from build123d import *

# Parameters (mm, degrees)
F1_DEPTH = 3.175


with BuildPart() as f1:
    # F0 (on Front) → F1 (new body)
    with BuildSketch(Plane.XZ):
        with BuildLine():
            Line((-26.0459613055, 0), (-8.255, 0))
            Line((-8.255, 0), (-8.255, 3.175))
            Line((-8.255, 3.175), (8.255, 3.175))
            Line((8.255, 3.175), (8.255, 0))
            Line((8.255, 0), (20.955, 0))
            add(Edge.make_bspline(
                [(20.955, 0), (20.9736007659, 4.7706959948), (21.0039408253, 12.5522680544), (24.2599950378, 16.0448016341), (25.5707021463, 17.3285181683)],
                knots=[0, 0, 0, 0, 0.5863679016, 0.9564357243, 0.9564357243, 0.9564357243, 0.9564357243], degree=3))
            ThreePointArc((25.5707021463, 17.3285181683), (25.9142071586, 17.8340267538), (26.035, 18.4331458679))
            Line((26.035, 18.4331458679), (26.035, 30.48))
            Line((26.035, 30.48), (22.8629365507, 30.48))
            Line((22.8629365507, 30.48), (22.8629365507, 46.9999574125))
            Line((22.8629365507, 46.9999574125), (26.035, 46.9999574125))
            Line((26.035, 46.9999574125), (26.035, 53.3499574125))
            Line((26.035, 53.3499574125), (19.6908731014, 53.3499574125))
            add(Edge.make_bspline(
                [(-26.0459613055, 6.35), (-14.6993313754, 12.8784414899), (6.7793902362, 25.2365229805), (15.5524054536, 44.3388670459), (19.6908731014, 53.3499574125)],
                knots=[0, 0, 0, 0, 0.5282730572, 1, 1, 1, 1], degree=3))
            Line((-26.0459613055, 6.35), (-26.0459613055, 0))
        make_face()
    extrude(amount=F1_DEPTH)


solid = f1.part
The model under review builds one solid part; all positions refer to its coordinate system, in mm. A direction names the side the tool comes from. Coordinates: 2 decimals unless noted, no trailing zeros.
(1) Insertion check: P1, Ø1.6, axis at x = -1.5, y = -1, coming from the -Z side (3 decimals); P2, Ø8, axis at x = -18.5, z = 13.5, coming from the +Y side; P3, Ø1, axis at y = -2, z = 39, coming from the +X side; P4, Ø1, axis at y = -1.5, z = 1, coming from the +X side. Each pin has a flat end and moves straight along its axis. Give the tip position at first contact, or say it passes through.
Determined:
P1: stops at z = 3.175
P2: stops at y = 0
P3: stops at x = 22.86
P4: stops at x = 20.96
(2) Draft analysis for pull direction Z (two halves, no side actions). For faces 1 (the flat face through (0, -2, 3.175)), 2 (the flat face through (24, -2, 47)), 3 (the flat face through (22.863, -2, 39)), 4 (the flat face through (8.255, -2, 2)), state which applies: +Z half, -Z half, draft (parallel to the pull), parting line (faces both ways), or undercut.
Determined:
face 1: -Z half
face 2: undercut
face 3: undercut
face 4: draft
(3) Tool access review of faces 5 (the flat face through (-17, -2, 0)), 6 (the flat face through (-8.255, -2, 2)), 7 (the flat face through (24, -2, 30.48)): name each direction out of +Z, -Z, +X, -X, +Y, -Y from which nothing blocks a thin tool from reaching the whole face with its end or side.
Determined:
face 5: -Z, +X, -X, +Y, -Y
face 6: -Z, +Y, -Y
face 7: +X, +Y, -Y
(4) Wall thickness on L1, parallel to X at y = -2.35, z = 2.5 (3 decimals); L2, parallel to X at y = -1.45, z = 18; L3, parallel to Z at x = -1.5, y = -2.45 (3 decimals): over which ranges is each line inside the solid? List them lowest first.
Determined:
L1: x = -26.046 to -8.255, 8.255 to 20.971
L2: x = -7.1 to 25.97
L3: z = 3.175 to 22.252
